from build123d import *

# Parameters (mm, degrees)
SKETCH1_R           = 47.5
SKETCH1_R_2         = 11
SKETCH1_R_3         = 1.5
BOSS_EXTRUDE1_DEPTH = 4.34
SKETCH2_R           = 28.7
SKETCH2_R_2         = 27.5
CUT_EXTRUDE1_DEPTH  = 2
CUT_EXTRUDE2_REACH  = 6.34
SKETCH3_R           = 2


with BuildPart() as part:
    # Sketch1 → Boss-Extrude1 (new body)
    with BuildSketch(Plane(origin=(0, 0, 0), x_dir=(1, 0, 0), z_dir=(0, 1, 0))):
        Circle(SKETCH1_R)
        Circle(SKETCH1_R_2, mode=Mode.SUBTRACT)
        with Locations((15.55, 15.55)):
            Circle(SKETCH1_R_3, mode=Mode.SUBTRACT)
        with Locations((15.55, -15.55)):
            Circle(SKETCH1_R_3, mode=Mode.SUBTRACT)
        with Locations((-15.55, -15.55)):
            Circle(SKETCH1_R_3, mode=Mode.SUBTRACT)
        with Locations((-15.55, 15.55)):
            Circle(SKETCH1_R_3, mode=Mode.SUBTRACT)
    extrude(amount=BOSS_EXTRUDE1_DEPTH)

    # Sketch2 → Cut-Extrude1 (cut)
    with BuildSketch(Plane(origin=(0, 4.34, 0), x_dir=(1, 0, 0), z_dir=(0, 1, 0))):
        Circle(SKETCH2_R)
        Circle(SKETCH2_R_2, mode=Mode.SUBTRACT)
    extrude(amount=-CUT_EXTRUDE1_DEPTH, mode=Mode.SUBTRACT)

    # Sketch3 → Cut-Extrude2 (cut, up to next)
    with BuildSketch(Plane(origin=(0, 4.34, 0), x_dir=(1, 0, 0), z_dir=(0, 1, 0)), mode=Mode.PRIVATE) as cut_extrude2_sk1:
        with Locations((24.04163056, 0)):
            Circle(SKETCH3_R)
    cut_extrude2_tool1 = extrude(cut_extrude2_sk1.sketch, amount=-CUT_EXTRUDE2_REACH, mode=Mode.PRIVATE) & part.part
    add(cut_extrude2_tool1.solids().sort_by_distance((24.041631, 4.34, 0))[0], mode=Mode.SUBTRACT)
    # Sketch3 → Cut-Extrude2 (cut, up to next)
    with BuildSketch(Plane(origin=(0, 4.34, 0), x_dir=(1, 0, 0), z_dir=(0, 1, 0)), mode=Mode.PRIVATE) as cut_extrude2_sk2:
        with Locations((0, -24.04163056)):
            Circle(SKETCH3_R)
    cut_extrude2_tool2 = extrude(cut_extrude2_sk2.sketch, amount=-CUT_EXTRUDE2_REACH, mode=Mode.PRIVATE) & part.part
    add(cut_extrude2_tool2.solids().sort_by_distance((0, 4.34, 24.041631))[0], mode=Mode.SUBTRACT)
    # Sketch3 → Cut-Extrude2 (cut, up to next)
    with BuildSketch(Plane(origin=(0, 4.34, 0), x_dir=(1, 0, 0), z_dir=(0, 1, 0)), mode=Mode.PRIVATE) as cut_extrude2_sk3:
        with Locations((-24.04163056, 0)):
            Circle(SKETCH3_R)
    cut_extrude2_tool3 = extrude(cut_extrude2_sk3.sketch, amount=-CUT_EXTRUDE2_REACH, mode=Mode.PRIVATE) & part.part
    add(cut_extrude2_tool3.solids().sort_by_distance((-24.041631, 4.34, 0))[0], mode=Mode.SUBTRACT)
    # Sketch3 → Cut-Extrude2 (cut, up to next)
    with BuildSketch(Plane(origin=(0, 4.34, 0), x_dir=(1, 0, 0), z_dir=(0, 1, 0)), mode=Mode.PRIVATE) as cut_extrude2_sk4:
        with Locations((0, 24.04163056)):
            Circle(SKETCH3_R)
    cut_extrude2_tool4 = extrude(cut_extrude2_sk4.sketch, amount=-CUT_EXTRUDE2_REACH, mode=Mode.PRIVATE) & part.part
    add(cut_extrude2_tool4.solids().sort_by_distance((0, 4.34, -24.041631))[0], mode=Mode.SUBTRACT)


solid = part.part
Could you check a few things on this model? Use its own coordinates, in mm. A direction names the side the tool comes from. Give positions to 0.01 mm unless a question says otherwise; leave off trailing zeros. Order: outer loops, then holes, each group sorted by start corner. A loop starts at its lowest first (then second) coordinate and runs counter-clockwise, first axis right, second up.
1. Suppose I cut it at A-A (z = 0). Write out the boundary of the cut face in (x, y), plus the area to 3 significant figures.
Answers below:
outline: (-47.5, 0) - (-26.04, 0) - (-26.04, 4.34) - (-27.5, 4.34) - (-27.5, 2.34) - (-28.7, 2.34) - (-28.7, 4.34) - (-47.5, 4.34) - close; (-22.04, 0) - (-11, 0) - (-11, 4.34) - (-22.04, 4.34) - close; (11, 0) - (22.04, 0) - (22.04, 4.34) - (11, 4.34) - close; (26.04, 0) - (47.5, 0) - (47.5, 4.34) - (28.7, 4.34) - (28.7, 2.34) - (27.5, 2.34) - (27.5, 4.34) - (26.04, 4.34) - close
area: 277 mm2
2. Suppose I cut it at B-B (x = -15.55). Write out the boundary of the cut face in (y, z).
Answers below:
outline: (0, -44.88) - (4.34, -44.88) - (4.34, -24.12) - (2.34, -24.12) - (2.34, -22.68) - (4.34, -22.68) - (4.34, -17.05) - (0, -17.05) - close; (0, -14.05) - (4.34, -14.05) - (4.34, 14.05) - (0, 14.05) - close; (0, 17.05) - (4.34, 17.05) - (4.34, 22.68) - (2.34, 22.68) - (2.34, 24.12) - (4.34, 24.12) - (4.34, 44.88) - (0, 44.88) - close
3. Thinking about a two-plate mould opening in X: for faces 3 (the cylindrical face through (-10.3, 2.14, 46.37)), 4 (the cylindrical face through (-15.875, 2.14, -14.086)), 5 (the flat face through (0, 4.34, 12)), 6 (the cylindrical face through (16.98, 2.14, 15.1)), which applies, +X half, -X half, draft (parallel to the pull), parting line (faces both ways), or undercut?
Answers below:
face 3: parting line
face 4: undercut
face 5: draft
face 6: undercut
4. I need wall thicknesses on L1, parallel to X at y = 1.8, z = 0; L2, parallel to Z at x = 0, y = 3.2. Which ranges of each line are inside material? Lowest first, please.
Answers below:
L1: x = -47.5 to -26.04, -22.04 to -11, 11 to 22.04, 26.04 to 47.5
L2: z = -47.5 to -28.7, -27.5 to -26.04, -22.04 to -11, 11 to 22.04, 26.04 to 27.5, 28.7 to 47.5
5. For pin 1 (2.5 mm diameter, centred on x = -15.55, z = -15.55, fed in from +Y); pin 2 (1.5 mm diameter, centred on y = 0.5, z = -6.5, fed in from -X), each with a flat end and sliding along its axis, tell me the tip position at first contact or that it passes through.
Answers below:
pin 1: passes through
pin 2: stops at x = -47.15
6. Suppose I cut it at C-C (z = -15.55). Write out the boundary of the cut face in (x, y).
Answers below:
outline: (-44.88, 0) - (-17.05, 0) - (-17.05, 4.34) - (-22.68, 4.34) - (-22.68, 2.34) - (-24.12, 2.34) - (-24.12, 4.34) - (-44.88, 4.34) - close; (-14.05, 0) - (14.05, 0) - (14.05, 4.34) - (-14.05, 4.34) - close; (17.05, 0) - (44.88, 0) - (44.88, 4.34) - (24.12, 4.34) - (24.12, 2.34) - (22.68, 2.34) - (22.68, 4.34) - (17.05, 4.34) - close
7. Suppose I cut it at D-D (y = 1.55). State how many separate pieces and enclosed holes the cut face has, plus the area to 3 significant figures.
Answers below:
separate pieces: 1
enclosed holes: 9
area: 6,630 mm2
8. Which directions (+Z, -Z, +X, -X, +Y, -Y) give clear straight access to the entire face, cutting with the end or side of a thin tool? Please do faces 1 (the cylindrical face through (15.43, 3.35, -24.2)), 2 (the cylindrical face through (-2.38, 2.14, 10.74)).
Answers below:
face 1: +Y
face 2: +Y, -Y
